Can you work these out from the model? Positions are in its coordinate system, mm. A direction names the side the tool comes from. Coordinates: 2 decimals unless noted, no trailing zeros. Order: outer loops, then holes, each group sorted by start corner. A loop starts at its lowest first (then second) coordinate and runs counter-clockwise, first axis right, second up. Notation, with made-up numbers: M 64.25,83 L 107.25,83 A25 cw 107.25,102 Z; hole C -31.5,23 d10. An arc over 180 degrees is marked long. Answer as a JSON object with one key per item and string values.
from build123d import *

# Parameters (mm, degrees)
BOSS_EXTRUDE1_DEPTH      = 254.000001
BOSS_EXTRUDE1_DEPTH_BACK = 254.000001
SKETCH3_W                = 50.8
SKETCH3_H                = 25.4
SKETCH3_W_2              = 47.625
SKETCH3_H_2              = 22.225
F_10_CLEARANCE_HOLE1_D   = 4.9784


with BuildPart() as part:
    # Sketch3 → Boss-Extrude1 (new, two sides: drawn at the far end of the back side and taken through both)
    with BuildSketch(Plane.XY.offset(-BOSS_EXTRUDE1_DEPTH_BACK)):
        Rectangle(SKETCH3_W, SKETCH3_H)
        Rectangle(SKETCH3_W_2, SKETCH3_H_2, mode=Mode.SUBTRACT)
    extrude(amount=BOSS_EXTRUDE1_DEPTH + BOSS_EXTRUDE1_DEPTH_BACK)

    # #10 Clearance Hole1 (through all)
    with Locations(Plane(origin=(25.4, 0, 0), x_dir=(0, 0, -1), z_dir=(1, 0, 0))):
        with Locations((-215.900000508, 0), (-241.261771093, 0), (215.899999492, 0), (241.261770077, -0.163454089)):
            Hole(F_10_CLEARANCE_HOLE1_D / 2)


solid = part.part
Item 1: Please list where these lines run through material, in increasing order: line 1 (Y direction, x = 11.5, z = -5); line 2 (X direction, y = -9, z = 78.5); line 3 (Y direction, x = -25, z = -215).
Answers follow:
{"line 1": "y = -12.7 to -11.11, 11.11 to 12.7", "line 2": "x = -25.4 to -23.81, 23.81 to 25.4", "line 3": "y = -12.7 to -2.32, 2.32 to 12.7"}
Item 2: If we mould it in two halves opening along Y, with no side actions, what happens to faces 3 (the flat face through (0, -11.112, -4)), 4 (the flat face through (0, 12.7, -4)), 5 (the flat face through (0, -12, -254)), 6 (the flat face through (0, 11.112, -4))? For each: pulls with the +Y half, pulls with the -Y half, needs draft (parallel to the pull), parting line crosses it, or undercut.
Answers follow:
{"face 3": "undercut", "face 4": "pulls with the +Y half", "face 5": "needs draft", "face 6": "undercut"}
Item 3: Which directions (+Z, -Z, +X, -X, +Y, -Y) give clear straight access to the entire face, cutting with the end or side of a thin tool? Please do faces 1 (the flat face through (0, -12, 254)), 2 (the flat face through (23.812, 0, -4)).
Answers follow:
{"face 1": "+Z, +X, -X, +Y, -Y", "face 2": "+Z, -Z"}
Item 4: I'm going to push a flat-ended pin straight in: pin 1 (4.5 mm diameter, centred on y = 0, z = 215.9, fed in from +X). Where does the tip first touch, or does it pass through?
Answers follow:
{"pin 1": "passes through"}
Item 5: I want a section at B-B, the plane z = 184.5. Write out the boundary of the cut face in (x, y), plus the area to 3 significant figures.
Answers follow:
{"outline": "M -25.4,-12.7 L 25.4,-12.7 L 25.4,12.7 L -25.4,12.7 Z; hole M -23.81,-11.11 L 23.81,-11.11 L 23.81,11.11 L -23.81,11.11 Z", "area": "232 mm^2"}
Item 6: I want a section at A-A, the plane x = -0.5. Write out the boundary of the cut face in (y, z), plus the area to 3 significant figures.
Answers follow:
{"outline": "M -12.7,-254 L -11.11,-254 L -11.11,254 L -12.7,254 Z; M 11.11,-254 L 12.7,-254 L 12.7,254 L 11.11,254 Z", "area": "1,610 mm^2"}
